Part model, mm, in its own coordinate system. Face numbers are marked on the shaded views. A direction names the side the tool comes from. Coordinates: 2 decimals unless noted, no trailing zeros. Loops run counter-clockwise (first coordinate to the right, second up) from the corner with the lowest first, then second, coordinate; pieces in that order, holes last. Notation, with made-up numbers: M 18,61.25 L 50,61.25 A9 ccw 50,72.25 Z; hole C 66.5,11.25 d7. An arc over 180 degrees is marked long. Use a Markdown table: item, result. Add a question column.
1) Band-saw the part on D-D (y = 3.25). List the corners of the cut face in (x, z) (3 decimals).
2) Band-saw the part on A-A (y = 16.5). List the corners of the cut face in (x, z).
3) Wall check: probe 1 along Z at (x, y) = (-18, 12.25); probe 2 along X at (y, z) = (10.5, -6); probe 3 along Z at (x, y) = (16.5, 6). Give the ranges that are in metal, low to high. Write a range as from..to.
4) Pin check, flat tips, straight feed: pin 1 Ø8 at (y, z) = (7, 24) entering from +X; pin 2 Ø7 at (x, z) = (-16.02, 9.25) entering from -Y; pin 3 Ø8 at (y, z) = (14.5, -7.5) entering from -X; pin 4 Ø12 at (x, z) = (3, 4) entering from +Y. Stop position of each tip, or through.
5) Tool access for the marked faces 1 and 2: list every direction of +Z, -Z, +X, -X, +Y, -Y with a clear straight run to the whole face (end or side of a thin tool).
6) Band-saw the part on B-B (z = 0). List the corners of the cut face in (x, y).
7) Band-saw the part on C-C (x = -1). List the corners of the cut face in (y, z).
8) Pull direction Z, two halves, no side cores. Call the marked faces 3, 4 and 5: released by +Z, released by -Z, zero draft, split by the parting line, or undercut.
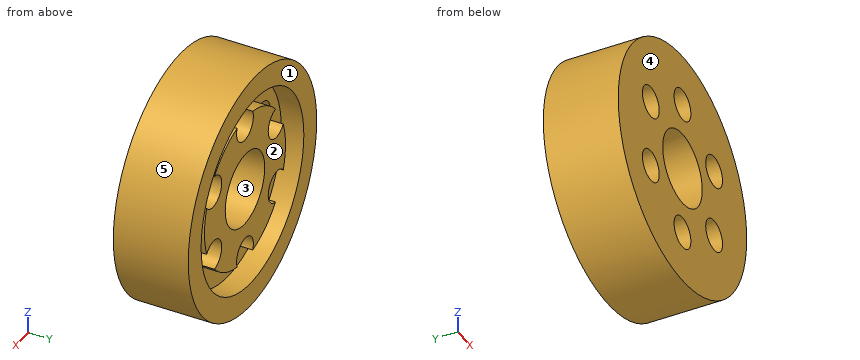
from build123d import *

# Parameters (mm, degrees)
SKETCH1_R           = 32.5
BOSS_EXTRUDE1_DEPTH = 20
SKETCH2_R           = 26
CUT_EXTRUDE1_DEPTH  = 6
SKETCH3_R           = 20.5
BOSS_EXTRUDE2_DEPTH = 4
SKETCH8_R           = 10
CUT_EXTRUDE2_DEPTH  = 21
CIRPATTERN1_COUNT   = 6


with BuildPart() as part:
    # Sketch1 → Boss-Extrude1 (new body)
    with BuildSketch(Plane(origin=(0, 0, 0), x_dir=(1, 0, 0), z_dir=(0, 1, 0))):
        Circle(SKETCH1_R)
    extrude(amount=BOSS_EXTRUDE1_DEPTH)

    # Sketch2 → Cut-Extrude1 (cut)
    with BuildSketch(Plane(origin=(0, 20, 0), x_dir=(1, 0, 0), z_dir=(0, 1, 0))):
        Circle(SKETCH2_R)
    extrude(amount=-CUT_EXTRUDE1_DEPTH, mode=Mode.SUBTRACT)

    # Sketch3 → Boss-Extrude2 (add)
    with BuildSketch(Plane(origin=(0, 14, 0), x_dir=(1, 0, 0), z_dir=(0, 1, 0))):
        Circle(SKETCH3_R)
    extrude(amount=BOSS_EXTRUDE2_DEPTH)

    # Sketch6 → M10 Tapped Hole1 (revolve, cut)
    with BuildSketch(Plane(origin=(0, 0, 18.5), x_dir=(0, 0, -1), z_dir=(1, 0, 0))):
        Polygon((0, 0), (0, 37.053657631), (4.25, 34.5), (4.25, 0), align=None)
    m10_tapped_hole1 = revolve(axis=Axis((0, -6.35, 18.5), (0, 1, 0)), mode=Mode.SUBTRACT)

    # Sketch8 → Cut-Extrude2 (cut, through all)
    with BuildSketch(Plane.XZ):
        Circle(SKETCH8_R)
    extrude(amount=-CUT_EXTRUDE2_DEPTH, mode=Mode.SUBTRACT)

    # CirPattern1: M10 Tapped Hole1 ×6 about axis
    cirpattern1_axis = Axis((0, 0, 0), (0, 1, 0))
    for i in range(1, CIRPATTERN1_COUNT):
        add(m10_tapped_hole1.rotate(cirpattern1_axis, i * 360 / CIRPATTERN1_COUNT), mode=Mode.SUBTRACT)


solid = part.part
Entries:
| question | item | result |
|---|---|---|
| 1 | outline | C 0,0 d65; hole C -16.021,-9.25 d8.5; hole C -16.021,9.25 d8.5; hole C 0,0 d20; hole C 0,-18.5 d8.5; hole C 0,18.5 d8.5; hole C 16.021,-9.25 d8.5; hole C 16.021,9.25 d8.5 |
| 2 | outline | C 0,0 d65; M -19.39,-6.66 A4.25 cw long -15.46,-13.46 A20.5 ccw -3.93,-20.12 A4.25 cw long 3.93,-20.12 A20.5 ccw 15.46,-13.46 A4.25 cw long 19.39,-6.66 A20.5 ccw 19.39,6.66 A4.25 cw long 15.46,13.46 A20.5 ccw 3.93,20.12 A4.25 cw long -3.93,20.12 A20.5 ccw -15.46,13.46 A4.25 cw long -19.39,6.66 A20.5 ccw Z; hole C 0,0 d52; hole C 0,0 d20 |
| 3 | probe 1 | -27.06..-13.01, -5.49..5.49, 13.01..27.06 |
| 3 | probe 2 | -31.94..-18.76, -13.28..-8, 8..13.28, 18.76..31.94 |
| 3 | probe 3 | -28..-13.47, -5.03..5.03, 13.47..28 |
| 4 | pin 1 | x = 25.62 |
| 4 | pin 2 | through |
| 4 | pin 3 | x = -32.31 |
| 4 | pin 4 | y = 18 |
| 5 | face 1 | +Z, -Z, +X, -X, +Y |
| 5 | face 2 | +Y |
| 6 | outline | M -32.5,0 L -10,0 L -10,18 L -20.5,18 L -20.5,14 L -26,14 L -26,20 L -32.5,20 Z; M 10,0 L 32.5,0 L 32.5,20 L 26,20 L 26,14 L 20.5,14 L 20.5,18 L 10,18 Z |
| 7 | outline | M 0,-32.48 L 20,-32.48 L 20,-25.98 L 14,-25.98 L 14,-22.63 L 0,-22.63 Z; M 0,-14.37 L 18,-14.37 L 18,-9.95 L 0,-9.95 Z; M 0,9.95 L 18,9.95 L 18,14.37 L 0,14.37 Z; M 0,22.63 L 14,22.63 L 14,25.98 L 20,25.98 L 20,32.48 L 0,32.48 Z |
| 8 | face 3 | undercut |
| 8 | face 4 | zero draft |
| 8 | face 5 | split by the parting line |
